Read the model definition and answer for the solid it produces. Units are mm, in the model's axes. A direction names the side the tool comes from. Round coordinates to 2 decimals unless told otherwise and drop trailing zeros. Answer as a JSON object with one key per item and string values. Group by question number.
Item 1: Given P1, Ø4, axis at x = -10, y = 2.5, coming from the +Z side; P2, Ø1, axis at y = -6, z = 5.5, coming from the +X side; P3, Ø1.5, axis at y = -1.5, z = 4, coming from the +X side; P4, Ø4, axis at x = -14.17, y = 0, coming from the -Z side, each flat-ended and moving along its own axis, determine where each tip first touches the part or whether it passes through.
Item 2: For faces 5 (the cylindrical face through (-12.54, -7.46, 2.72)), 6 (the flat face through (0, 0, 6.35)), 7 (the cylindrical face through (-12.54, 7.48, 2.7)), determine the directions among +Z, -Z, +X, -X, +Y, -Y from which every point of the face is accessible in a straight line to the end or side of a thin tool.
Item 3: The mould has two halves that part along X. Classify faces 1 (the flat face through (-12, -2, 3.175)), 2 (the cylindrical face through (-18.6, -7.46, 0.8)), 3 (the cylindrical face through (-16, 1.7, 1.6)), 4 (the flat face through (-4.98, 0.11, 3.22)): pulls with the +X half, pulls with the -X half, needs draft (parallel to the pull), parting line crosses it, or undercut.
Item 4: Consider probe 1 along Y at (x, z) = (14, 1); probe 2 along Z at (x, y) = (1, 0.25) (3 decimals); probe 3 along Z at (x, y) = (9.5, -5) (3 decimals). Determine where each line is inside the solid, lowest interval first. Write a range as from..to.
Item 5: Section A-A, the plane y = 0 is taken. Count the separate pieces of the cut face and the enclosed holes in it, plus the area to 3 significant figures.
from build123d import *

# Parameters (mm, degrees)
F4_R     = 2.5
F5_DEPTH = 3.175
F6_R     = 1.5875


with BuildPart() as f3:
    # F3: sweep along a path in F0
    with BuildLine(Plane.XZ) as f3_path:
        Line((-19.05, 0), (-6.8411742094, 0))
        Line((-6.8411742094, 0), (-3.175, 6.35))
        Line((-3.175, 6.35), (0, 6.35))
        Line((0, 6.35), (3.175, 6.35))
        Line((3.175, 6.35), (6.8411742094, 0))
        Line((6.8411742094, 0), (19.05, 0))
    # F2 (on line) → F3 (sweep)
    with BuildSketch(Plane(origin=(-19.05, 0, 0), x_dir=(0, -1, 0), z_dir=(-1, 0, 0))):
        with BuildLine():
            Line((-7.9375, 0), (7.9375, 0))
            Line((7.9375, 0), (7.9375, 1.5875))
            ThreePointArc((7.9375, 1.5875), (7.4725320151, 2.7100320151), (6.35, 3.175))
            Line((6.35, 3.175), (-6.35, 3.175))
            ThreePointArc((-6.35, 3.175), (-7.4725320151, 2.7100320151), (-7.9375, 1.5875))
            Line((-7.9375, 1.5875), (-7.9375, 0))
        make_face()
    sweep(path=f3_path.line, transition=Transition.RIGHT)

    # F4 (on face) → F5 (cut, through all)
    with BuildSketch(Plane.XY.offset(3.175)):
        with Locations((-14.16875, 0)):
            Circle(F4_R)
        with Locations((14.16875, 0)):
            Circle(F4_R)
    extrude(amount=-F5_DEPTH, mode=Mode.SUBTRACT)

    # F6
    f6_edges = [f3.edges().sort_by_distance(p)[0] for p in [
        (-19.05, 0, 3.175),
        (19.05, 0, 3.175),
    ]]
    fillet(f6_edges, radius=F6_R)


solid = f3.part
Values found:
{
 "1": {"P1": "z = 4.34", "P2": "x = 7.62", "P3": "x = 8.63", "P4": "through"},
 "2": {"face 5": "+Z, -X, -Y", "face 6": "-Z, +Y, -Y", "face 7": "+Z, -X, +Y"},
 "3": {"face 1": "needs draft", "face 2": "pulls with the -X half", "face 3": "undercut", "face 4": "undercut"},
 "4": {"probe 1": "-7.94..-2.49, 2.49..7.94", "probe 2": "6.35..9.525", "probe 3": "0..3.175"},
 "5": {"separate pieces": "3", "enclosed holes": "0", "area": "111 mm2"}
}
